```python
from build123d import *

# Parameters (mm, degrees)
SKETCH2_W           = 170
SKETCH2_H           = 185
BOSS_EXTRUDE1_DEPTH = 9.8
SKETCH4_R           = 3
SKETCH4_R_2         = 2.5
SKETCH4_R_3         = 20
SKETCH4_R_4         = 9
SKETCH4_R_5         = 13
SKETCH4_R_6         = 10
SKETCH4_R_7         = 2.75
SKETCH4_R_8         = 11
SKETCH4_R_9         = 12.5
SKETCH4_W           = 20
SKETCH4_H           = 185
SKETCH4_H_2         = 35
SKETCH4_H_3         = 50
HOLES_DEPTH         = 9.8
FEET_DEPTH          = 23
SKETCH7_R           = 3
FEET_HOLE_DEPTH     = 10
MOTOR_SINK_START    = -9.8
SKETCH9_R           = 6
MOTOR_SINK_DEPTH    = 4
BOSS_EXTRUDE2_DEPTH = 0.2
FILLET4_R           = 10
CUT_EXTRUDE2_DEPTH  = 129.534392285
FILLET6_R           = 2
CUT_EXTRUDE3_DEPTH  = 198.296325359
FILLET7_R           = 5


# Some blends are built 0.0001 mm under size
with BuildPart() as part:
    # Sketch2 → Boss-Extrude1 (new body)
    with BuildSketch(Plane.XY):
        Rectangle(SKETCH2_W, SKETCH2_H)
    extrude(amount=-BOSS_EXTRUDE1_DEPTH)

    # Sketch4 → holes (cut)
    with BuildSketch(Plane.XY):
        with Locations((50, 77.5)):
            Circle(SKETCH4_R)
        with Locations(Location((50, -72.5, 0), (0, 0, 180))):
            Circle(SKETCH4_R)
        with Locations(Location((-25, -22.5, 0), (0, 0, 180))):
            Circle(SKETCH4_R_2)
        with Locations((-50, 77.5)):
            Circle(SKETCH4_R)
        with Locations((50, 2.5)):
            Circle(SKETCH4_R_3)
        with Locations(Location((25, -22.5, 0), (0, 0, 180))):
            Circle(SKETCH4_R)
        with Locations((-50, 62.5)):
            Circle(SKETCH4_R)
        with Locations(Location((-25, 27.5, 0), (0, 0, 180))):
            Circle(SKETCH4_R_2)
        with Locations((0, 2.5)):
            Circle(SKETCH4_R_3)
        with Locations((0, 35.804729394)):
            Circle(SKETCH4_R)
        with Locations((0, -30.804729394)):
            Circle(SKETCH4_R)
        with Locations(Location((75, -22.5, 0), (0, 0, 180))):
            Circle(SKETCH4_R)
        with Locations(Location((75, 27.5, 0), (0, 0, 180))):
            Circle(SKETCH4_R)
        with Locations(Location((25, 27.5, 0), (0, 0, 180))):
            Circle(SKETCH4_R)
        with Locations(Location((35, -72.5, 0), (0, 0, 180))):
            Circle(SKETCH4_R)
        with Locations(Location((-50, -30.804729394, 0), (0, 0, 180))):
            Circle(SKETCH4_R)
        with Locations(Location((-20, 77.5, 0), (0, 0, 180))):
            Circle(SKETCH4_R)
        with Locations((20, 77.5)):
            Circle(SKETCH4_R)
        with Locations(Location((-50, 35.804729394, 0), (0, 0, 180))):
            Circle(SKETCH4_R)
        with Locations((-44.446789408, 17.751552332)):
            Circle(SKETCH4_R_4)
        with Locations((0, 61.5)):
            Circle(SKETCH4_R_5)
        with Locations((-46.819261128, -11.562260058)):
            Circle(SKETCH4_R_6)
        with Locations((-35, -72.5)):
            Circle(SKETCH4_R)
        with Locations((-33.304729394, 2.5)):
            Circle(SKETCH4_R_7)
        with Locations((35, -50)):
            Circle(SKETCH4_R_8)
        with Locations((-40, -52.5)):
            Circle(SKETCH4_R_9)
        with Locations(Location((-50, -72.5, 0), (0, 0, 180))):
            Circle(SKETCH4_R)
        with Locations(Location((-35, 62.5, 0), (0, 0, 180))):
            Circle(SKETCH4_R)
        with Locations(Location((-35, 52.5, 0), (0, 0, 180))):
            Circle(SKETCH4_R)
        with Locations((50, -30.804729394)):
            Circle(SKETCH4_R)
        with Locations((35, 77.5)):
            Circle(SKETCH4_R)
        with Locations(Location((-35, 77.5, 0), (0, 0, 180))):
            Circle(SKETCH4_R)
        with Locations((65, -50)):
            Circle(SKETCH4_R_8)
        with Locations(Location((50, 62.5, 0), (0, 0, 180))):
            Circle(SKETCH4_R)
        with Locations((50, 35.804729394)):
            Circle(SKETCH4_R)
        with Locations(Location((65, -72.5, 0), (0, 0, 180))):
            Circle(SKETCH4_R)
        with Locations(Location((80, -72.5, 0), (0, 0, 180))):
            Circle(SKETCH4_R)
        with Locations((-50, 52.5)):
            Circle(SKETCH4_R)
        with Locations((35, 62.5)):
            Circle(SKETCH4_R)
        with Locations(Location((-20, 52.5, 0), (0, 0, 180))):
            Circle(SKETCH4_R)
        with Locations((20, 52.5)):
            Circle(SKETCH4_R)
        with Locations(Location((-20, 62.5, 0), (0, 0, 180))):
            Circle(SKETCH4_R)
        with Locations((20, 62.5)):
            Circle(SKETCH4_R)
        with Locations((35, 52.5)):
            Circle(SKETCH4_R)
        with Locations(Location((50, 52.5, 0), (0, 0, 180))):
            Circle(SKETCH4_R)
        with Locations((-75, 0)):
            Rectangle(SKETCH4_W, SKETCH4_H)
        with Locations((0, -65)):
            Rectangle(SKETCH4_W, SKETCH4_H_2)
        with Locations((75, 67.5)):
            Rectangle(SKETCH4_W, SKETCH4_H_3)
    extrude(amount=-HOLES_DEPTH, mode=Mode.SUBTRACT)

    # Sketch6 → feet (add)
    with BuildSketch(Plane(origin=(0, 0, -9.8), x_dir=(-1, 0, 0), z_dir=(0, 0, -1))):
        Polygon((-10, -82.5), (-10, -92.5), (-85, -92.5), (-85, -82.5), (-18, -82.5), (-18, -42.5), (-10, -42.5), align=None)
        Polygon((10, -82.5), (10, -42.5), (18, -42.5), (18, -82.5), (65, -82.5), (65, -92.5), (10, -92.5), align=None)
    extrude(amount=FEET_DEPTH)

    # Sketch7 → feet-hole (cut)
    with BuildSketch(Plane.XZ.offset(92.5)):
        with Locations((60, -25)):
            Circle(SKETCH7_R)
        with Locations((30, -25)):
            Circle(SKETCH7_R)
        with Locations((-30, -25)):
            Circle(SKETCH7_R)
        with Locations((-60, -25)):
            Circle(SKETCH7_R)
    extrude(amount=-FEET_HOLE_DEPTH, mode=Mode.SUBTRACT)

    # Sketch9 → motor_sink (cut)
    with BuildSketch(Plane(origin=(0, 0, -9.8), x_dir=(-1, 0, 0), z_dir=(0, 0, -1)).offset(MOTOR_SINK_START)):
        with Locations((-75, -22.5)):
            Circle(SKETCH9_R)
        with Locations((-25, -22.5)):
            Circle(SKETCH9_R)
        with Locations((-25, 27.5)):
            Circle(SKETCH9_R)
        with Locations((-75, 27.5)):
            Circle(SKETCH9_R)
        with Locations((-50, -30.804729394)):
            Circle(SKETCH9_R)
        with Locations((25, 27.5)):
            Circle(SKETCH9_R)
        with Locations((25, -22.5)):
            Circle(SKETCH9_R)
        with Locations((0, -30.804729394)):
            Circle(SKETCH9_R)
        with Locations((-50, 35.804729394)):
            Circle(SKETCH9_R)
        with Locations((33.304729394, 2.5)):
            Circle(SKETCH9_R)
        with Locations((0, 35.804729394)):
            Circle(SKETCH9_R)
    extrude(amount=MOTOR_SINK_DEPTH, mode=Mode.SUBTRACT)

    # Sketch13 → Boss-Extrude2 (add)
    with BuildSketch(Plane.XY):
        Polygon((-65, 92.5), (65, 92.5), (65, 42.5), (85, 42.5), (85, -92.5), (-65, -92.5), align=None)
    extrude(amount=BOSS_EXTRUDE2_DEPTH)

    # Fillet4
    fillet4_edges = [part.edges().sort_by_distance(p)[0] for p in [
        (65, 42.5, -4.8),
        (-65, 92.5, -4.8),
        (85, 42.5, -4.8),
        (65, 92.5, -4.8),
    ]]
    fillet(fillet4_edges, radius=FILLET4_R - 0.0001)  # a hair under: the kernel refuses the full size

    # Sketch14 → Cut-Extrude2 (cut, through all)
    with BuildSketch(Plane(origin=(18, 0, 0), x_dir=(0, 0, -1), z_dir=(1, 0, 0))):
        Polygon((32.8, -82.5), (9.8, -42.5), (32.8, -42.5), align=None)
    extrude(amount=-CUT_EXTRUDE2_DEPTH, mode=Mode.SUBTRACT)

    # Fillet6
    fillet6_edges = [part.edges().sort_by_distance(p)[0] for p in [
        (14, -42.5, -9.8),
        (51.5, -82.5, -9.8),
        (-41.5, -82.5, -9.8),
        (-14, -42.5, -9.8),
    ]]
    fillet(fillet6_edges, radius=FILLET6_R)

    # Sketch16 → Cut-Extrude3 (cut, through all)
    with BuildSketch(Plane(origin=(0, -82.5, 0), x_dir=(1, 0, 0), z_dir=(0, 1, 0))):
        Polygon((85, 11.8), (64, 32.8), (85, 32.8), align=None)
    extrude(amount=-CUT_EXTRUDE3_DEPTH, mode=Mode.SUBTRACT)

    # Fillet7
    # the kernel refuses this fillet: 5 mm, written as the material it takes off along each edge
    with BuildSketch(Plane(origin=(85, -77.32233047, -11.8), x_dir=(0, 0, 1), z_dir=(0, -1, 0))) as fillet7_piece_1:
        with BuildLine():
            CenterArc((FILLET7_R * 0.414213562373, FILLET7_R), FILLET7_R, 225, 45)
            Line((-FILLET7_R * 0.292893218813, FILLET7_R * 0.292893218813), (0, 0))
            Line((0, 0), (FILLET7_R * 0.414213562373, 0))
        make_face()
    extrude(amount=20.355339059, mode=Mode.SUBTRACT)
    with BuildSketch(Plane(origin=(64, -77.32233047, -32.8), x_dir=(-1, 0, 0), z_dir=(0, -1, 0))) as fillet7_piece_2:
        with BuildLine():
            CenterArc((FILLET7_R * 0.414213562373, -FILLET7_R), FILLET7_R, 90, 45)
            Line((-FILLET7_R * 0.292893218813, -FILLET7_R * 0.292893218813), (0, 0))
            Line((0, 0), (FILLET7_R * 0.414213562373, 0))
        make_face()
    extrude(amount=20.355339059, mode=Mode.SUBTRACT)
    with BuildSketch(Plane(origin=(-65, -70, -32.8), x_dir=(0, 0, 1), z_dir=(0, -1, 0))) as fillet7_piece_3:
        with BuildLine():
            CenterArc((FILLET7_R, -FILLET7_R), FILLET7_R, 90, 90)
            Line((0, -FILLET7_R), (0, 0))
            Line((0, 0), (FILLET7_R, 0))
        make_face()
    extrude(amount=35, mode=Mode.SUBTRACT)


solid = part.part
```
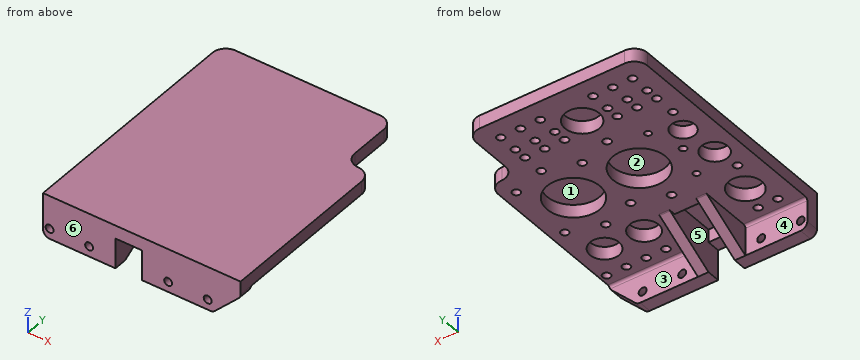
Work out the finished part from the listing and answer in its coordinate system (mm). Face numbers are marked on the shaded views. A direction names the side the tool comes from. Give positions to 0.01 mm unless a question says otherwise; leave off trailing zeros. Write each loop counter-clockwise with the first axis right and the second up, starting at its lowest first coordinate (ties: lowest second). Pieces come first, ordered by that corner, then holes. Notation, with made-up numbers: (21, 43) - (63, 43) arc R28 cw to (63, 81) - close; hole circle Ø3 at (20.5, 48). An arc over 180 degrees is marked (long way). Use one line per item in the form item = value.
1. Consider L1, parallel to Y at x = 0, z = -5; L2, parallel to Z at x = 71, y = -21; L3, parallel to Y at x = -25, z = -2. Determine where each line is inside the solid, lowest interval first.
Filled in:
L1 = -92.5 to -82.5, -47.5 to -33.8, -27.8 to -17.5, 22.5 to 32.8, 38.8 to 48.5, 74.5 to 92.5
L2 = -9.8 to -4, 0 to 0.2
L3 = -92.5 to -28.5, -16.5 to 21.5, 33.5 to 92.5
2. For the marked faces 4, 5 and 6, determine the directions among +Z, -Z, +X, -X, +Y, -Y from which every point of the face is accessible in a straight line to the end or side of a thin tool.
Filled in:
face_4 = -Z, -X, +Y
face_5 = -Z
face_6 = +Z, -Z, +X, -X, -Y
3. A cutting plane is placed at B-B (x = 60). Write down the section's boundary in (y, z).
Filled in:
outline = (-92.5, -32.8) - (-82.5, -32.8) - (-82.5, -28) - (-92.5, -28) - close; (-92.5, -22) - (-82.5, -22) - (-82.5, -11.8) arc R2 cw to (-80.5, -9.8) - (-59.8, -9.8) - (-59.8, 0) - (-40.2, 0) - (-40.2, -9.8) - (-14.82, -9.8) - (-14.82, 0) - (19.82, 0) - (19.82, -9.8) - (91.16, -9.8) - (91.16, 0.2) - (-92.5, 0.2) - close
4. Each of these flat-tipped pins is pushed along its axis until it touches: pin 1 Ø5 at (x, z) = (13, -23.5) entering from +Y; pin 2 Ø8 at (x, y) = (35, -47) entering from -Z; pin 3 Ø5 at (x, y) = (49, 63.5) entering from -Z. Where does it stop, or does it pass through?
Filled in:
pin_1 = -61.98
pin_2 = 0
pin_3 = -9.8
5. Determine the mould class of the marked faces 1, 2 and 3 for opening direction X: released by +X, released by -X, zero draft, split by the parting line, or undercut.
Filled in:
face_1 = undercut
face_2 = undercut
face_3 = zero draft
6. A cutting plane is placed at A-A (z = -17). Write down the section's boundary in (x, y), and give its area (3 significant figures).
Filled in:
outline = (-65, -92.5) - (-10, -92.5) - (-10, -55.02) - (-18, -55.02) - (-18, -82.5) - (-65, -82.5) - close; (10, -92.5) - (79.8, -92.5) - (79.8, -82.5) - (18, -82.5) - (18, -55.02) - (10, -55.02) - close
area = 1,690 mm^2
